Read the model definition and answer for the solid it produces. Units are mm, in the model's axes. A direction names the side the tool comes from. Coordinates: 2 decimals unless noted, no trailing zeros. Order: outer loops, then holes, each group sorted by start corner. A loop starts at its lowest first (then second) coordinate and runs counter-clockwise, first axis right, second up. Notation, with made-up numbers: (85, -18) -> (104, -18) arc R22 cw to (104, -6) -> close; hole circle Ø8 at (-18, -29). An arc over 180 degrees is marked (long way). Answer as a JSON object with one key per item and string values. Group by question number.
1) Given pin 1 (2 mm diameter, centred on y = -3.5, z = 7.5, fed in from -X); pin 2 (1.5 mm diameter, centred on y = 19, z = 0.5, fed in from -X), each flat-ended and moving along its own axis, determine where each tip first touches the part or whether it passes through.
2) Section B-B on y = 6 is taken. Determine the outline of the cut face in (x, z) (3 decimals).
3) Determine the mould class of faces 3 (the cylindrical face through (-13.458, 11.394, 0.178)), 4 (the cylindrical face through (1.61, 30.417, -0.099)), 5 (the cylindrical face through (-16.631, -10.526, 0.178)), 6 (the flat face through (0, 19, 0)) for opening direction X: released by +X, released by -X, zero draft, split by the parting line, or undercut.
4) Section C-C on x = -16.5 is taken. Determine the outline of the cut face in (y, z).
5) Consider L1, parallel to X at y = 0, z = 6.25 (3 decimals); L2, parallel to Y at x = -18.25, z = -10.5; L3, parallel to X at y = 31.5, z = 10 (3 decimals). Determine where each line is inside the solid, lowest interval first.
6) A tool of negligible diameter and unlimited length cuts with its end or side. For faces 1 (the cylindrical face through (-12.94, 9.2, 0.18)), 2 (the flat face through (1, 5, 12.7)), from which of +Z, -Z, +X, -X, +Y, -Y can it reach the whole face along a straight path? Write none if from no direction.
from build123d import *

# Parameters (mm, degrees)
F1_DEPTH = 12.7
F2_R     = 1.58749
F3_R     = 1.5875
F5_D     = 4.4958


# Not quite as in the source:
# - a fillet or chamfer is up to 0.001 mm smaller than in the source, because OpenCascade refuses the exact size


with BuildPart() as f1:
    # F0 (on Top) → F1 (new body, symmetric)
    with BuildSketch(Plane.XY):
        with BuildLine():
            Line((0, 37.6967221242), (0, 0))
            ThreePointArc((0, 0), (-15.024261314, -7.7771299333), (-12.7, 8.9802561211))
            Line((-12.7, 8.9802561211), (-12.7, 12.2967221242))
            ThreePointArc((-12.7, 12.2967221242), (-17.3021299333, -10.040231571), (3.175, 0))
            Line((3.175, 0), (3.175, 37.6967221242))
            Line((3.175, 37.6967221242), (0, 37.6967221242))
        make_face()
    extrude(amount=F1_DEPTH, both=True)

    # F2 (radius 1.5875 in the source; OpenCascade refuses exactly that, so slightly less here)
    f2_edges = [f1.edges().sort_by_distance(p)[0] for p in [
        (-12.7, 8.980256, 0),
        (-12.7, 12.296722, 0),
    ]]
    fillet(f2_edges, radius=F2_R)

    # F3
    f3_edges = [f1.edges().sort_by_distance(p)[0] for p in [
        (1.5875, 37.696722, 12.7),
        (1.5875, 37.696722, -12.7),
    ]]
    fillet(f3_edges, radius=F3_R)

    # F5 (through all)
    with Locations(Plane(origin=(0, 0, 0), x_dir=(0, 1, 0), z_dir=(-1, 0, 0))):
        with Locations((28.1717221242, 0)):
            Hole(F5_D / 2)


solid = f1.part
Worked answers:
{
 "1": {"pin 1": "stops at x = -21.98", "pin 2": "stops at x = 0"},
 "2": {"outline": "(-20.718, -12.7) -> (-16.923, -12.7) -> (-16.923, 12.7) -> (-20.718, 12.7) -> close; (0, -12.7) -> (3.175, -12.7) -> (3.175, 12.7) -> (0, 12.7) -> close"},
 "3": {"face 3": "undercut", "face 4": "zero draft", "face 5": "split by the parting line", "face 6": "undercut"},
 "4": {"outline": "(-10.61, -12.7) -> (-6.49, -12.7) -> (-6.49, 12.7) -> (-10.61, 12.7) -> close; (6.49, -12.7) -> (10.61, -12.7) -> (10.61, 12.7) -> (6.49, 12.7) -> close"},
 "5": {"L1": "x = -22.225 to -19.05, 0 to 3.175", "L2": "y = -9.23 to -3.82, 3.82 to 9.23", "L3": "x = 0 to 3.175"},
 "6": {"face 1": "+Z, -Z", "face 2": "+Z, +X, -X, +Y, -Y"}
}
